from build123d import *

# Parameters (mm, degrees)
BOSS_EXTRUDE1_DEPTH                            = 4
SKETCH3_R                                      = 2.15
BOSS_EXTRUDE2_DEPTH                            = 8
BOSS_EXTRUDE3_START                            = -8
BOSS_EXTRUDE3_DEPTH                            = 8
CBORE_FOR_6_SOCKET_HEAD_CAP_SCREW1_D           = 3.6576
CBORE_FOR_6_SOCKET_HEAD_CAP_SCREW1_CBORE_D     = 7.14502
CBORE_FOR_6_SOCKET_HEAD_CAP_SCREW1_CBORE_DEPTH = 3.5052
BOSS_EXTRUDE5_DEPTH                            = 15
BOSS_EXTRUDE6_DEPTH                            = 5.75
CUT_EXTRUDE1_DEPTH                             = 49.104053883
CUT_EXTRUDE1_DEPTH_BACK                        = 20
SKETCH11_5_R                                   = 2.25
CUT_EXTRUDE2_DEPTH                             = 6.1
CHAMFER2_SIZE                                  = 10
SKETCH18_R                                     = 2
BOSS_EXTRUDE10_DEPTH                           = 2
CHAMFER3_SIZE                                  = 5
CHAMFER3_SIZE2                                 = 0.881634904
BOSS_EXTRUDE7_DEPTH                            = 4
BOSS_EXTRUDE9_DEPTH                            = 8


with BuildPart() as part:
    # Sketch2 → Boss-Extrude1 (new body)
    with BuildSketch(Plane.XY):
        with BuildLine():
            Line((1, 0), (20, 0))
            Line((20, 0), (20, 27))
            Line((20, 27), (1, 27))
            ThreePointArc((1, 27), (0.292893219, 26.707106781), (0, 26))
            Line((0, 26), (0, 1))
            ThreePointArc((0, 1), (0.292893219, 0.292893219), (1, 0))
        make_face()
    extrude(amount=BOSS_EXTRUDE1_DEPTH)

    # Sketch3 → Boss-Extrude2 (add)
    with BuildSketch(Plane.XY):
        with Locations((4.5, 22.5)):
            Circle(SKETCH3_R)
        with Locations((4.5, 4.5)):
            Circle(SKETCH3_R)
    extrude(amount=-BOSS_EXTRUDE2_DEPTH)

    # Sketch3<3> → Boss-Extrude3 (add)
    with BuildSketch(Plane.XY.offset(BOSS_EXTRUDE3_START)):
        with BuildLine():
            Line((4.5, 15), (4.5, 12))
            ThreePointArc((4.5, 12), (8.782801805, 10.656915518), (11.531693039, 7.108695652))
            ThreePointArc((11.531693039, 7.108695652), (12.997768364, 5.216311724), (15.281929326, 4.5))
            Line((15.281929326, 4.5), (20, 4.5))
            Line((20, 4.5), (20, 27))
            Line((20, 27), (12, 27))
            Line((12, 27), (12, 22.5))
            ThreePointArc((12, 22.5), (9.803300859, 17.196699141), (4.5, 15))
        make_face()
    extrude(amount=BOSS_EXTRUDE3_DEPTH)

    # CBORE for #6 Socket Head Cap Screw1 (through all)
    with Locations(Plane.XY.offset(4)):
        with Locations((13.5, 13.5)):
            CounterBoreHole(CBORE_FOR_6_SOCKET_HEAD_CAP_SCREW1_D / 2, CBORE_FOR_6_SOCKET_HEAD_CAP_SCREW1_CBORE_D / 2, CBORE_FOR_6_SOCKET_HEAD_CAP_SCREW1_CBORE_DEPTH)

    # Sketch11 → Boss-Extrude5 (add)
    with BuildSketch(Plane(origin=(0, 27, 0), x_dir=(1, 0, 0), z_dir=(0, 1, 0))):
        Polygon((12, 8), (12, -4), (35, -4), (39, 2), (39, 8), align=None)
    extrude(amount=BOSS_EXTRUDE5_DEPTH)

    # Sketch13 → Boss-Extrude6 (add)
    with BuildSketch(Plane(origin=(0, 10.25, 0), x_dir=(-1, 0, 0), z_dir=(0, -1, 0))):
        Polygon((-20, -4), (-20, 8), (-39, 8), (-39, 2), (-35, -4), align=None)
    extrude(amount=BOSS_EXTRUDE6_DEPTH)

    # Sketch11<5> → Cut-Extrude1 (cut, two sides: drawn at the far end of the back side and taken through both)
    with BuildSketch(Plane(origin=(0, 27, 0), x_dir=(1, 0, 0), z_dir=(0, 1, 0)).offset(-CUT_EXTRUDE1_DEPTH_BACK)):
        with Locations((32.5, 8)):
            Circle(SKETCH11_5_R)
    extrude(amount=CUT_EXTRUDE1_DEPTH + CUT_EXTRUDE1_DEPTH_BACK, mode=Mode.SUBTRACT)

    # Sketch14 → Cut-Extrude2 (cut)
    with BuildSketch(Plane(origin=(0, 32, 0), x_dir=(-1, 0, 0), z_dir=(0, -1, 0))):
        with BuildLine():
            Line((-29.85, 14.55), (-29.85, 1.45))
            Line((-29.85, 1.45), (-28.547785431, 1.45))
            ThreePointArc((-28.547785431, 1.45), (-25.8382832, 4.239145141), (-24.85, 8))
            ThreePointArc((-24.85, 8), (-25.8382832, 11.760854859), (-28.547785431, 14.55))
            Line((-28.547785431, 14.55), (-29.85, 14.55))
        make_face()
        with BuildLine():
            Line((-28.547785431, 1.45), (-29.85, 1.45))
            Line((-29.85, 1.45), (-29.85, 14.55))
            Line((-29.85, 14.55), (-28.547785431, 14.55))
            ThreePointArc((-28.547785431, 14.55), (-40.15, 8), (-28.547785431, 1.45))
        make_face()
        with BuildLine():
            ThreePointArc((-24.85, 8), (-25.8382832, 4.239145141), (-28.547785431, 1.45))
            Line((-28.547785431, 1.45), (-24.85, 1.45))
            Line((-24.85, 1.45), (-24.85, 8))
        make_face()
        Polygon((-24.85, 8), (-24.85, 1.45), (-9.85, 1.45), (-9.85, 14.55), (-24.85, 14.55), align=None)
        with BuildLine():
            Line((-24.85, 14.55), (-28.547785431, 14.55))
            ThreePointArc((-28.547785431, 14.55), (-25.8382832, 11.760854859), (-24.85, 8))
            Line((-24.85, 8), (-24.85, 14.55))
        make_face()
    extrude(amount=-CUT_EXTRUDE2_DEPTH, mode=Mode.SUBTRACT)

    # Chamfer2
    chamfer2_edges = [part.edges().sort_by_distance(p)[0] for p in [
        (12, 42, -2),
    ]]
    chamfer(chamfer2_edges, length=CHAMFER2_SIZE)

    # Sketch18 → Boss-Extrude10 (add)
    with BuildSketch(Plane(origin=(0, 0, -8), x_dir=(-1, 0, 0), z_dir=(0, 0, -1))):
        with Locations(Location((-16, 26, 0), (0, 0, 180))):
            Circle(SKETCH18_R)
    extrude(amount=BOSS_EXTRUDE10_DEPTH)

    # Chamfer3
    chamfer3_edges = [part.edges().sort_by_distance(p)[0] for p in [
        (20, 18.625, 4),
    ]]
    chamfer3_side = [part.faces().sort_by_distance(p)[0] for p in [
        (20, 18.625, -2),
    ]]
    chamfer(chamfer3_edges, length=CHAMFER3_SIZE, length2=CHAMFER3_SIZE2, reference=chamfer3_side[0])

    # Sketch15 → Boss-Extrude7 (add)
    with BuildSketch(Plane.XY.offset(4)):
        Polygon((20, 4.5), (20, 0), (13.07179677, 0), (20, -4), (31, -4), (35, 0), (35, 4.5), align=None)
    extrude(amount=-BOSS_EXTRUDE7_DEPTH)

    # Sketch17 → Boss-Extrude9 (add)
    with BuildSketch(Plane(origin=(0, 0, 0), x_dir=(-1, 0, 0), z_dir=(0, 0, -1))):
        with BuildLine():
            Line((-30.25, 0), (-15.870834875, 0))
            ThreePointArc((-15.870834875, 0), (-15.146390506, -0.555885716), (-15.495834875, -1.399519053))
            Line((-15.495834875, -1.399519053), (-20, -4))
            Line((-20, -4), (-31, -4))
            Line((-31, -4), (-31, -0.75))
            ThreePointArc((-31, -0.75), (-30.780330086, -0.219669914), (-30.25, 0))
        make_face()
    extrude(amount=BOSS_EXTRUDE9_DEPTH)


solid = part.part
Geometry: final body of the model. Coordinates: model frame, mm. A direction names the side the tool comes from. Coordinates: 2 decimals unless noted, no trailing zeros. Loops run counter-clockwise (first coordinate to the right, second up) from the corner with the lowest first, then second, coordinate; pieces in that order, holes last. Notation, with made-up numbers: (20.5, 55.25) - (24.5, 55.25) arc R19 ccw to (24.5, 66.25) - close; hole circle Ø7 at (-31, -11.5). An arc over 180 degrees is marked (long way). One line per question, with ' | ' between items. Start each with the question number.
(1) First-contact query: pin 1 (8 mm diameter, centred on y = 33.5, z = -7.5, fed in from -X); pin 2 (6 mm diameter, centred on x = 8.5, z = -7, fed in from -Y); pin 3 (4.5 mm diameter, centred on x = 21.5, y = 39, fed in from -Z); pin 4 (8 mm diameter, centred on x = 26.5, y = 17.5, fed in from -Z). Flat tips, straight axial feed; report the tip coordinate or a pass-through.
(2) Cut plane D-D on y = 28.5. Output: boundary loops of the cut face in (x, z), and give its area (3 significant figures).
(3) Ray query, L1, parallel to Y at x = 26.5, z = -5; L2, parallel to Y at x = 33.5, z = -3.25; L3, parallel to Z at x = 24, y = 31. Return the intervals inside material, ascending. Write a range as from..to.
(4) Draft query along Y for faces 5 (the flat face through (4, 5, -8)), 6 (the flat face through (18, 38, -1)), 7 (the flat face through (33, -2, 2)), 8 (the flat face through (29, 38.1, -4)). Return one class per face: +Y half, -Y half, draft (parallel to the pull), parting line (faces both ways), or undercut.
(5) Reachability of faces 1 (the flat face through (20, 19, -5)), 2 (the cylindrical face through (34.371, 35.007, -0.582)), 3 (the flat face through (23, -2, -8)), 4 (the flat face through (22, 35, -1.45)) from +Z, -Z, +X, -X, +Y, -Y: full face, straight path, thin tool, end or side. Return the list, or none.
(6) Cut plane A-A on x = 32.5. Output: boundary loops of the cut face in (y, z), and give its area (3 significant figures).
(7) Cut plane C-C on x = 26.5. Output: boundary loops of the cut face in (y, z).
(8) Cut plane B-B on y = 9. Output: boundary loops of the cut face in (x, z).
Here are the results:
1) pin 1: x = 12 | pin 2: y = 2.6 | pin 3: z = -8 | pin 4: through
2) outline: (12, -8) - (30.25, -8) arc R2.25 cw to (34.75, -8) - (39, -8) - (39, -2) - (35, 4) - (12, 4) - close | area: 304 mm²
3) L1: -4..0, 4.5..10.25, 27..32, 38.1..42 | L2: 4.5..10.25, 27..32, 38.1..42 | L3: -8..4
4) face 5: draft | face 6: +Y half | face 7: -Y half | face 8: undercut
5) face 1: +Z, -Z, +X | face 2: -Z | face 3: -Z, +X, -X, -Y | face 4: -Z, -X
6) outline: (-2.5, 0) - (4.5, 0) - (4.5, -8) - (7, -8) - (7, -5.75) - (10.25, -5.75) - (10.25, 4) - (-2.5, 4) - close; (27, -5.75) - (32, -5.75) - (32, -0.35) - (38.1, -0.35) - (38.1, -5.75) - (42, -5.75) - (42, 4) - (27, 4) - close | area: 203 mm²
7) outline: (-4, -8) - (0, -8) - (0, 0) - (4.5, 0) - (4.5, -8) - (10.25, -8) - (10.25, 4) - (-4, 4) - close; (27, -8) - (32, -8) - (32, -1.45) - (38.1, -1.45) - (38.1, -8) - (42, -8) - (42, 4) - (27, 4) - close
8) outline: (0, 0) - (10.5, 0) - (10.5, -8) - (30.25, -8) arc R2.25 cw to (34.75, -8) - (39, -8) - (39, -2) - (35, 4) - (0, 4) - close
